CAD build for the part. Positions are in the model's coordinates, mm. A direction names the side the tool comes from. Give positions to 0.01 mm unless a question says otherwise; leave off trailing zeros. Order: outer loops, then holes, each group sorted by start corner. A loop starts at its lowest first (then second) coordinate and runs counter-clockwise, first axis right, second up. Notation, with made-up numbers: (5.25, 53.25) -> (61.25, 53.25) arc R22 ccw to (61.25, 86.25) -> close; hole circle Ø11 at (51, 34.25). An arc over 180 degrees is marked (long way). Answer as CSV lines item,"result".
```python
from build123d import *

# Parameters (mm, degrees)
F0_R     = 8.25
F1_DEPTH = 56.2
F3_DEPTH = 25
F4_DEPTH = 25
F6_DEPTH = 25
F7_DEPTH = 10.5
F8_DEPTH = 25
F9_DEPTH = 25


with BuildPart() as f1:
    # F0 (on Front) → F1 (new body)
    with BuildSketch(Plane.XZ):
        Circle(F0_R)
    extrude(amount=F1_DEPTH)

    # F2 (on face) → F3 (join)
    with BuildSketch(Plane.XZ.offset(56.2)):
        with BuildLine():
            Line((-13.0284968764, -8.25), (0, -8.25))
            ThreePointArc((0, -8.25), (-8.25, 0), (0, 8.25))
            Line((0, 8.25), (0, 34.5139689744))
            Line((0, 34.5139689744), (-13.0284968764, 34.5139689744))
            Line((-13.0284968764, 34.5139689744), (-13.0284968764, -8.25))
        make_face()
    extrude(amount=F3_DEPTH)

    # F2 (on face) → F4 (join)
    with BuildSketch(Plane.XZ.offset(56.2)):
        with BuildLine():
            ThreePointArc((8.25, 0), (5.8336309448, -5.8336309448), (0, -8.25))
            Line((0, -8.25), (13.0284968764, -8.25))
            Line((13.0284968764, -8.25), (13.0284968764, 34.5139689744))
            Line((13.0284968764, 34.5139689744), (0, 34.5139689744))
            Line((0, 34.5139689744), (0, 8.25))
            ThreePointArc((0, 8.25), (5.8336309448, 5.8336309448), (8.25, 0))
        make_face()
    extrude(amount=F4_DEPTH)

    # F5 (on face) → F6 (join)
    with BuildSketch(Plane.XZ.offset(81.2)):
        Polygon((-13.0284968764, 0), (-13.0284968764, 34.5139689744), (-121.5313971043, 91.8013229966), (-121.5313971043, 57.2873540223), align=None)
    extrude(amount=-F6_DEPTH)

    # F7 (add): faces of the model
    f7_faces = [f1.faces().sort_by_distance(p)[0] for p in [
        (-6.5142484382, -68.7, -8.25),
        (6.5142484382, -68.7, -8.25),
    ]]
    extrude(f7_faces, amount=F7_DEPTH)

    # F8 (add): a face of the model
    f8_faces = [f1.faces().sort_by_distance(p)[0] for p in [
        (0, -56.2, 0),
    ]]
    extrude(f8_faces, amount=F8_DEPTH)

    # F9 (add): a face of the model
    f9_faces = [f1.faces().sort_by_distance(p)[0] for p in [
        (0, 0, 0),
    ]]
    extrude(f9_faces, amount=F9_DEPTH)


solid = f1.part
```
1) Band-saw the part on C-C, the plane y = -16. Write the cut outline in (x, z).
Data:
outline,"circle Ø16.5 at (0, 0)"
2) Band-saw the part on A-A, the plane x = 0. Write the cut outline in (y, z).
Data:
outline,"(-81.2, -18.75) -> (-56.2, -18.75) -> (-56.2, -8.25) -> (25, -8.25) -> (25, 8.25) -> (-56.2, 8.25) -> (-56.2, 34.51) -> (-81.2, 34.51) -> close"
3) Band-saw the part on D-D, the plane z = 16. Write the cut outline in (x, y).
Data:
outline,"(-43.33, -81.2) -> (13.03, -81.2) -> (13.03, -56.2) -> (-43.33, -56.2) -> close"
4) Which spindle directions (+Z, -Z, +X, -X, +Y, -Y) get a long thin tool onto all of the face, cutting with end or side? Do faces 1 (the flat face through (-13.028, -69, -9)), 2 (the flat face through (0, -69, 34.514)), 3 (the flat face through (-50, -81.2, 41)). Say none if no direction does.
Data:
face 1,"-Z, -X, +Y, -Y"
face 2,"+Z, +X, +Y, -Y"
face 3,"+Z, -Z, +X, -X, -Y"
5) Pin check, flat tip, straight feed: P1, Ø20, axis at x = -3, y = -74.5, coming from the +Z side. Stop position of the tip, or through.
Data:
P1,"stops at z = 34.51"
6) Wall check: line 1 along Y through (x, z) = (-44, 20.5); line 2 along X through (y, z) = (-69, -3); line 3 along X through (y, z) = (-60.5, 3). Give the ranges that are in metal, low to high. Write a range as [from, to].
Data:
line 1,"y = [-81.2, -56.2]"
line 2,"x = [-13.03, 13.03]"
line 3,"x = [-18.71, 13.03]"
7) Band-saw the part on B-B, the plane z = 4. Write the cut outline in (x, y), then the cut area to 3 significant figures.
Data:
outline,"(-20.6, -81.2) -> (13.03, -81.2) -> (13.03, -56.2) -> (7.22, -56.2) -> (7.22, 25) -> (-7.22, 25) -> (-7.22, -56.2) -> (-20.6, -56.2) -> close"
area,"2,010 mm2"
